```python
from build123d import *

# Parameters (mm, degrees)
SKETCH1_W           = 50
SKETCH1_H           = 65
BOSS_EXTRUDE1_DEPTH = 3
SKETCH2_W           = 3
SKETCH2_H           = 65
BOSS_EXTRUDE2_DEPTH = 25
SKETCH4_R           = 12.499228858
CUT_EXTRUDE1_DEPTH  = 3
SKETCH5_R           = 2
CUT_EXTRUDE2_DEPTH  = 30


with BuildPart() as part:
    # Sketch1 → Boss-Extrude1 (new body)
    with BuildSketch(Plane(origin=(0, 0, 0), x_dir=(1, 0, 0), z_dir=(0, 1, 0))):
        Rectangle(SKETCH1_W, SKETCH1_H)
    extrude(amount=BOSS_EXTRUDE1_DEPTH)

    # Sketch2 → Boss-Extrude2 (add)
    with BuildSketch(Plane(origin=(0, 3, 0), x_dir=(1, 0, 0), z_dir=(0, 1, 0))):
        with Locations((23.5, 0)):
            Rectangle(SKETCH2_W, SKETCH2_H)
    extrude(amount=BOSS_EXTRUDE2_DEPTH)

    # Sketch4 → Cut-Extrude1 (cut)
    with BuildSketch(Plane.XZ):
        with Locations(Location((0, 0, 0), (0, 0, 270))):
            Circle(SKETCH4_R)
    extrude(amount=-CUT_EXTRUDE1_DEPTH, mode=Mode.SUBTRACT)

    # Sketch5 → Cut-Extrude2 (cut)
    with BuildSketch(Plane.ZY.offset(-22)):
        with Locations((28.5, 10)):
            Circle(SKETCH5_R)
        with Locations((-28.5, 10)):
            Circle(SKETCH5_R)
    extrude(amount=-CUT_EXTRUDE2_DEPTH, mode=Mode.SUBTRACT)


solid = part.part
```
Could you check a few things on this model? Use its own coordinates, in mm. A direction names the side the tool comes from. Coordinates: 2 decimals unless noted, no trailing zeros. Write each loop counter-clockwise with the first axis right and the second up, starting at its lowest first coordinate (ties: lowest second). Pieces come first, ordered by that corner, then holes. Notation, with made-up numbers: M -19.75,36 L -6.75,36 A27 cw -6.75,62 Z; hole C 85.5,16 d11. An arc over 180 degrees is marked long. Answer as CSV lines item,"result". Start each with the question number.
1) Please list where these lines run through material, in increasing order: line 1 (Y direction, x = 23.45, z = 28.5); line 2 (Y direction, x = 14.5, z = 10.5); line 3 (X direction, y = 4.5, z = 9). Write a range as from..to.
2) I want a section at C-C, the plane y = 10. Please give me the cut outline in (x, z), and give its area (3 significant figures).
3) I want a section at A-A, the plane x = 0. Please give me the cut outline in (y, z), and give its area (3 significant figures).
4) I want a section at B-B, the plane z = 0. Please give me the cut outline in (x, y).
5) For faces 4 (the flat face through (-12, 3, -8)), 5 (the flat face through (-11, 0, -8)), which set-ups out of +Z, -Z, +X, -X, +Y, -Y let a thin tool reach every point of the face, with its end or its side?
6) We'd pull the mould along Z, two halves only. Please class faces 1 (the flat face through (25, 14, 0)), 2 (the flat face through (9.1, 2.5, -32.5)), 3 (the cylindrical face through (3.754, 1.479, -11.922)): +Z half, -Z half, draft (parallel to the pull), parting line (faces both ways), or undercut.
7) I want a section at D-D, the plane z = 19.5. Please give me the cut outline in (x, y), and give its area (3 significant figures).
8) For P1, Ø6, axis at y = 18.5, z = 16.5, coming from the -X side; P2, Ø3.5, axis at y = 10, z = 28.5, coming from the +X side; P3, Ø8, axis at x = -15.5, z = -23, coming from the +Y side, each with a flat end and sliding along its axis, tell me the tip position at first contact or that it passes through.
Data:
1,line 1,"y = 0..8, 12..28"
1,line 2,"y = 0..3"
1,line 3,"x = 22..25"
2,outline,"M 22,-32.5 L 25,-32.5 L 25,-30.5 L 22,-30.5 Z; M 22,-26.5 L 25,-26.5 L 25,26.5 L 22,26.5 Z; M 22,30.5 L 25,30.5 L 25,32.5 L 22,32.5 Z"
2,area,"171 mm^2"
3,outline,"M 0,-32.5 L 3,-32.5 L 3,-12.5 L 0,-12.5 Z; M 0,12.5 L 3,12.5 L 3,32.5 L 0,32.5 Z"
3,area,"120 mm^2"
4,outline,"M -25,0 L -12.5,0 L -12.5,3 L -25,3 Z; M 12.5,0 L 25,0 L 25,28 L 22,28 L 22,3 L 12.5,3 Z"
5,face 4,"+Z, -Z, -X, +Y"
5,face 5,"+Z, -Z, +X, -X, -Y"
6,face 1,"draft"
6,face 2,"-Z half"
6,face 3,"undercut"
7,outline,"M -25,0 L 25,0 L 25,28 L 22,28 L 22,3 L -25,3 Z"
7,area,"225 mm^2"
8,P1,"stops at x = 22"
8,P2,"passes through"
8,P3,"stops at y = 3"
